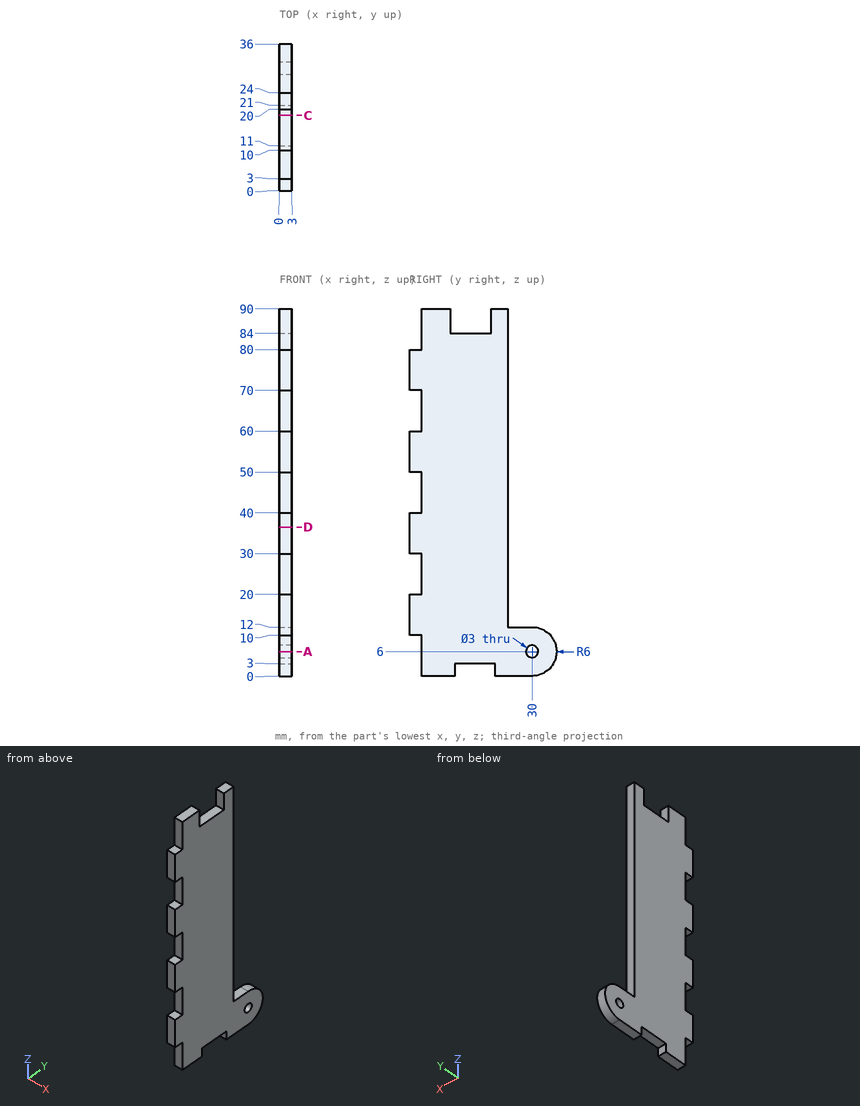
Part print with two shaded views. Sizes in mm from the minimum x, y, z corner. Give positions to 0.01 mm unless a question says otherwise; leave off trailing zeros. Order: outer loops, then holes, each group sorted by start corner. A loop starts at its lowest first (then second) coordinate and runs counter-clockwise, first axis right, second up. Notation, with made-up numbers: M -9.75,-8 L 21.25,-8 A29 ccw 21.25,14 Z; hole C -4.5,82.5 d11. An arc over 180 degrees is marked long. Write item = value, one per line.
Q1. Cut at C-C, the plane y = 18.5. List the corners of the cut face in (x, z).
Derived:
outline = M 0,3 L 3,3 L 3,84 L 0,84 Z
Q2. Flat gauge pins, fed straight in: pin 1 (1.5 mm diameter, centred on x = 2, z = 43.5, fed in from +Y); pin 2 (0.9 mm diameter, centred on x = 2, y = 1.5, fed in from +Z); pin 3 (1.5 mm diameter, centred on x = 2, y = 2, fed in from -Z). Where does each tip first touch, or does it go through?
Derived:
pin_1 = 24
pin_2 = 80
pin_3 = 10
Q3. Cut at D-D, the plane z = 36.5. List the corners of the cut face in (x, y), then the cut area to 3 significant figures.
Derived:
outline = M 0,0 L 3,0 L 3,24 L 0,24 Z
area = 72.0 mm2
Q4. Drill centre lines: line 1 (Z direction, x = 1.6, y = 2); line 2 (Y direction, x = 1.35, z = 6); line 3 (Y direction, x = 1.55, z = 25). Where is each one in solid material? Low to high. Write a range as [from, to].
Derived:
line_1 = [10, 20], [30, 40], [50, 60], [70, 80]
line_2 = [3, 28.5], [31.5, 36]
line_3 = [3, 24]
Q5. Cut at A-A, the plane z = 6. List the corners of the cut face in (x, y).
Derived:
outline = M 0,3 L 3,3 L 3,28.5 L 0,28.5 Z; M 0,31.5 L 3,31.5 L 3,36 L 0,36 Z
